```python
from build123d import *

# Parameters (mm, degrees)
SKETCH1_W           = 14.2
SKETCH1_H           = 5.4
BOSS_EXTRUDE1_DEPTH = 9.2
SKETCH2_W           = 0.5
SKETCH2_H           = 0.25
BOSS_EXTRUDE2_DEPTH = 3.5


with BuildPart() as part:
    # Sketch1 → Boss-Extrude1 (new body)
    with BuildSketch(Plane.XY):
        with Locations((7.1, 2.7)):
            Rectangle(SKETCH1_W, SKETCH1_H)
    extrude(amount=BOSS_EXTRUDE1_DEPTH)

    # Sketch2 → Boss-Extrude2 (add)
    with BuildSketch(Plane.XZ):
        with Locations((1.832645657, 8.389413507)):
            Rectangle(SKETCH2_W, SKETCH2_H)
        with Locations((4.466322828, 8.389413507)):
            Rectangle(SKETCH2_W, SKETCH2_H)
        with Locations((7.1, 8.389413507)):
            Rectangle(SKETCH2_W, SKETCH2_H)
        with Locations((9.733677172, 8.389413507)):
            Rectangle(SKETCH2_W, SKETCH2_H)
        with Locations((12.367354343, 8.389413507)):
            Rectangle(SKETCH2_W, SKETCH2_H)
        with Locations((4.466322828, 0.810586493)):
            Rectangle(SKETCH2_W, SKETCH2_H)
        with Locations((7.1, 0.810586493)):
            Rectangle(SKETCH2_W, SKETCH2_H)
        with Locations((9.733677172, 0.810586493)):
            Rectangle(SKETCH2_W, SKETCH2_H)
        with Locations((12.367354343, 0.810586493)):
            Rectangle(SKETCH2_W, SKETCH2_H)
        with Locations((1.832645657, 0.810586493)):
            Rectangle(SKETCH2_W, SKETCH2_H)
    extrude(amount=BOSS_EXTRUDE2_DEPTH)


solid = part.part
```
Source: CAD feature listing. Evaluate the final solid. Frame: model axes, mm. Round coordinates to 2 decimals unless told otherwise and drop trailing zeros. Loops run counter-clockwise (first coordinate to the right, second up) from the corner with the lowest first, then second, coordinate; pieces in that order, holes last.
1. Contact query for flat-ended pins moving along their axis: pin 1 (0.6 mm diameter, centred on x = 9.5, y = -1, fed in from +Z); pin 2 (0.6 mm diameter, centred on x = 12.5, y = -1, fed in from -Z); pin 3 (3 mm diameter, centred on y = 3.5, z = 4, fed in from -X). Output: stop coordinate, or through.
2. Section query C-C on z = 2.25. Output: boundary loops of the cut face in (x, y).
3. Section query A-A on y = -1.5. Give the number of separate pieces and of enclosed holes in the cut face, and give its area (3 significant figures).
4. Ray query, L1, parallel to Y at x = 8.25, z = 2.25. Return the intervals inside material, ascending.
5. Section query B-B on x = 1.25. Output: boundary loops of the cut face in (y, z), and give its area (3 significant figures).
Answers below:
1. pin 1: stops at z = 8.51
1. pin 2: stops at z = 0.69
1. pin 3: stops at x = 0
2. outline: (0, 0) - (14.2, 0) - (14.2, 5.4) - (0, 5.4) - close
3. separate pieces: 10
3. enclosed holes: 0
3. area: 1.25 mm2
4. L1: y = 0 to 5.4
5. outline: (0, 0) - (5.4, 0) - (5.4, 9.2) - (0, 9.2) - close
5. area: 49.7 mm2
